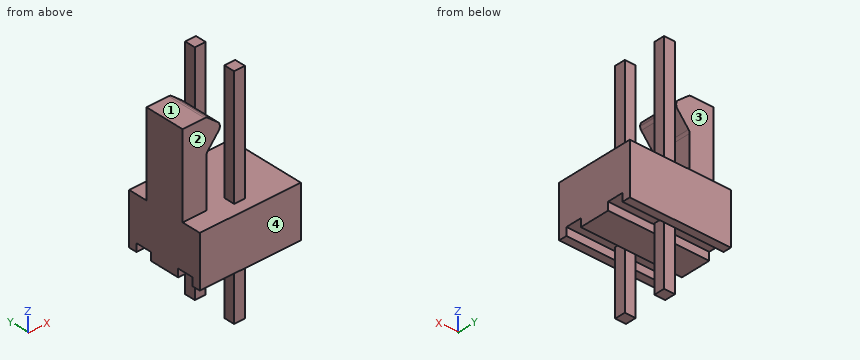
Solid Edge part; units mm, degrees
sketch "Sketch1" plane through (0, 0, 0) normal (0, -1, 0) x (1, 0, 0)
  line L0 (-3.17, -1.61) -> (3.17, -1.61)
  line L1 (3.17, -1.61) -> (3.17, 1.61)
  line L2 (3.17, 1.61) -> (-3.17, 1.61)
  line L3 (-3.17, 1.61) -> (-3.17, -1.61)
extrude "Protrusion1" add sketch "Sketch1" along normal mid plane 4.9
sketch "Sketch2" plane through (0, 0, 1.61) normal (0, 0, 1) x (1, 0, 0)
  line L0 (-3.17, -1.25) -> (-0.83, -1.25)
  line L1 (-0.83, -1.25) -> (-0.83, 1.25)
  line L2 (-0.83, 1.25) -> (-3.17, 1.25)
  line L3 (-3.17, 1.25) -> (-3.17, -1.25)
  dimension "D1" = 0.83
extrude "ExtrudedProtrusion_2" add sketch "Sketch2" along normal blind 5.2 and the other way blind 1.7629
sketch "Sketch3" plane through (3.17, 0, 0) normal (1, 0, 0) x (0, 1, 0)
  line L0 (-1.95, -1.11) -> (-0.95, -1.11)
  line L1 (-0.95, -1.11) -> (-0.95, -1.61)
  line L2 (-0.95, -1.61) -> (-1.95, -1.61)
  line L3 (-1.95, -1.61) -> (-1.95, -1.11)
  line L4 (1.95, -1.11) -> (0.95, -1.11)
  line L5 (0.95, -1.11) -> (0.95, -1.61)
  line L6 (0.95, -1.61) -> (1.95, -1.61)
  line L7 (1.95, -1.61) -> (1.95, -1.11)
  dimension "D1" = 1.95
  dimension "D2" = 1.95
extrude "Cutout1" cut sketch "Sketch3" against normal up to surface (6.34 mm away)
sketch "Sketch4" plane through (0, 0, 1.61) normal (0, 0, 1) x (0, 1, 0)
  line L0 (-1.7, -0.34) -> (-1.02, -0.34)
  line L1 (-1.02, -0.34) -> (-1.02, 0.34)
  line L2 (-1.02, 0.34) -> (-1.7, 0.34)
  line L3 (-1.7, 0.34) -> (-1.7, -0.34)
  line L4 (1.7, -0.34) -> (1.02, -0.34)
  line L5 (1.02, -0.34) -> (1.02, 0.34)
  line L6 (1.02, 0.34) -> (1.7, 0.34)
  line L7 (1.7, 0.34) -> (1.7, -0.34)
  dimension "D1" = 1.02
  dimension "D2" = 1.02
  dimension "D3" = 1.7
extrude "ExtrudedProtrusion_3" add sketch "Sketch4" along normal blind 7.4 and the other way blind 6.7
sketch "Sketch5" plane through (-2, 1.25, 4.21) normal (0, 1, 0) x (-1, 0, 0)
  line L0 (-0.33, 2.6) -> (-1.17, 2.6)
  line L1 (-1.17, 2.6) -> (-1.17, 1.907)
  line L2 (-1.17, 1.907) -> (-0.33, 2.6)
  line L3 (-0.33, 0.5827) -> (-1.17, 1.6008)
  line L4 (-1.17, 1.6008) -> (-1.17, -2.6)
  line L5 (-1.17, -2.6) -> (-0.33, -2.6)
  line L6 (-0.33, -2.6) -> (-0.33, 0.5827)
extrude "Cutout2" cut sketch "Sketch5" against normal up to surface (2.5 mm away)
fillet "Round_1" radius 0.3 4 edges at (-0.83, 0, 6.117) (-1.67, 0, 6.81) (-0.83, 0, 5.8108) (-1.67, 0, 4.7927)
Source: CAD feature listing. Evaluate the final solid. Frame: model axes, mm. Face numbers are marked on the shaded views. A direction names the side the tool comes from. Give positions to 0.01 mm unless a question says otherwise; leave off trailing zeros. Write each loop counter-clockwise with the first axis right and the second up, starting at its lowest first coordinate (ties: lowest second). Pieces come first, ordered by that corner, then holes. Notation, with made-up numbers: M -13.5,-7.75 L -2.5,-7.75 A24 ccw -2.5,27.25 Z; hole C -8,4 d7. An arc over 180 degrees is marked long. Answer as a JSON object with one key per item and string values.
Q1. Cut plane C-C, the plane y = 0.1. Return the cut outline in (x, z), then the cut area to 3 significant figures.
Geometry check:
{"outline": "M -3.17,-1.61 L 3.17,-1.61 L 3.17,1.61 L -1.67,1.61 L -1.67,4.68 A0.3 cw -1.6,4.88 L -0.9,5.73 A0.3 ccw -0.83,5.92 L -0.83,5.98 A0.3 ccw -0.94,6.21 L -1.59,6.74 A0.3 ccw -1.78,6.81 L -3.17,6.81 Z", "area": "29.2 mm^2"}
Q2. Cut plane A-A, the plane z = -1.25. Return the cut outline in (x, y).
Geometry check:
{"outline": "M -3.17,-2.45 L 3.17,-2.45 L 3.17,-1.95 L -3.17,-1.95 Z; M -3.17,-0.95 L 3.17,-0.95 L 3.17,0.95 L -3.17,0.95 Z; M -3.17,1.95 L 3.17,1.95 L 3.17,2.45 L -3.17,2.45 Z; M -0.34,-1.7 L 0.34,-1.7 L 0.34,-1.02 L -0.34,-1.02 Z; M -0.34,1.02 L 0.34,1.02 L 0.34,1.7 L -0.34,1.7 Z"}
Q3. Ray query, line 1 along Y through (x, z) = (0.25, 2); line 2 along X through (y, z) = (1.05, 3.75); line 3 along Z through (x, y) = (2.75, 1.7). Return the intervals inside material, ascending.
Geometry check:
{"line 1": "y = -1.7 to -1.02, 1.02 to 1.7", "line 2": "x = -3.17 to -1.67, -0.34 to 0.34", "line 3": "z = -1.11 to 1.61"}
Q4. Contact query for flat-ended pins moving along their axis: P1, Ø0.7, axis at x = 0, z = 6.5, coming from the +Y side; P2, Ø1.2, axis at x = -1.5, z = 4.5, coming from the -Y side; P3, Ø3, axis at x = 2.5, z = 3.5, coming from the -Y side; P4, Ø2.5, axis at x = -2.5, z = 4.5, coming from the +Y side. Output: stop coordinate, or through.
Geometry check:
{"P1": "stops at y = 1.7", "P2": "stops at y = -1.25", "P3": "passes through", "P4": "stops at y = 1.25"}
Q5. Access query for the marked faces 1, 2, 3 and 4. Directions: +Z, -Z, +X, -X, +Y, -Y. A direction counts if a zero-diameter tool reaches every point of the face in a straight line with its end or side. Return the directions, or none.
Geometry check:
{"face 1": "+Z, -X, +Y, -Y", "face 2": "+Z, -X, -Y", "face 3": "+Z, -X, +Y", "face 4": "+Z, -Z, +X, -X, -Y"}
Q6. Cut plane D-D, the plane z = 6.5. Return the cut outline in (x, y).
Geometry check:
{"outline": "M -3.17,-1.25 L -1.29,-1.25 L -1.29,1.25 L -3.17,1.25 Z; M -0.34,-1.7 L 0.34,-1.7 L 0.34,-1.02 L -0.34,-1.02 Z; M -0.34,1.02 L 0.34,1.02 L 0.34,1.7 L -0.34,1.7 Z"}
Q7. Cut plane B-B, the plane x = -2.5. Return the cut outline in (y, z).
Geometry check:
{"outline": "M -2.45,-1.61 L -1.95,-1.61 L -1.95,-1.11 L -0.95,-1.11 L -0.95,-1.61 L 0.95,-1.61 L 0.95,-1.11 L 1.95,-1.11 L 1.95,-1.61 L 2.45,-1.61 L 2.45,1.61 L 1.25,1.61 L 1.25,6.81 L -1.25,6.81 L -1.25,1.61 L -2.45,1.61 Z"}
